Geometry: final body of the model. Coordinates: model frame, mm. A direction names the side the tool comes from. Coordinates: 2 decimals unless noted, no trailing zeros. Order: outer loops, then holes, each group sorted by start corner. A loop starts at its lowest first (then second) coordinate and runs counter-clockwise, first axis right, second up. Notation, with made-up numbers: M -3.75,34.5 L 10.25,34.5 A16 ccw 10.25,62.5 Z; hole C -15,-12 d7. An arc over 180 degrees is marked long. One line per question, with ' | ' between items.
from build123d import *

# Parameters (mm, degrees)
BOSS_EXTRUDE2_DEPTH = 40
SKETCH4_R           = 12
CUT_EXTRUDE4_DEPTH  = 2
SKETCH5_R           = 6
CUT_EXTRUDE5_DEPTH  = 77.576758876
SKETCH6_R           = 3.4
CUT_EXTRUDE6_DEPTH  = 76.498344353
SKETCH7_R           = 3.4
CUT_EXTRUDE7_DEPTH  = 87.394444266


with BuildPart() as part:
    # Sketch1 → Boss-Extrude2 (new body)
    with BuildSketch(Plane(origin=(0, 0, 0), x_dir=(0, 0, -1), z_dir=(1, 0, 0))):
        Polygon((0, 0), (-50, 0), (-50, 18), (0, 18), (0, 58), (14, 58), (14, 0), align=None)
    extrude(amount=BOSS_EXTRUDE2_DEPTH)

    # Sketch4 → Cut-Extrude4 (cut)
    with BuildSketch(Plane(origin=(0, 18, 0), x_dir=(1, 0, 0), z_dir=(0, 1, 0))):
        with Locations(Location((20, -25, 0), (0, 0, 270))):
            Circle(SKETCH4_R)
    extrude(amount=-CUT_EXTRUDE4_DEPTH, mode=Mode.SUBTRACT)

    # Sketch5 → Cut-Extrude5 (cut, through all)
    with BuildSketch(Plane(origin=(0, 16, 0), x_dir=(1, 0, 0), z_dir=(0, 1, 0))):
        with Locations(Location((20, -25, 0), (0, 0, 270))):
            Circle(SKETCH5_R)
    extrude(amount=-CUT_EXTRUDE5_DEPTH, mode=Mode.SUBTRACT)

    # Sketch6 → Cut-Extrude6 (cut, through all)
    with BuildSketch(Plane(origin=(0, 18, 0), x_dir=(1, 0, 0), z_dir=(0, 1, 0))):
        with Locations(Location((20, -9, 0), (0, 0, 270))):
            Circle(SKETCH6_R)
        with Locations(Location((36, -25, 0), (0, 0, 270))):
            Circle(SKETCH6_R)
        with Locations(Location((20, -41, 0), (0, 0, 270))):
            Circle(SKETCH6_R)
        with Locations(Location((4, -25, 0), (0, 0, 270))):
            Circle(SKETCH6_R)
    extrude(amount=-CUT_EXTRUDE6_DEPTH, mode=Mode.SUBTRACT)

    # Sketch7 → Cut-Extrude7 (cut, through all)
    with BuildSketch(Plane.XY):
        with Locations((20, 47)):
            Circle(SKETCH7_R)
        with Locations((32, 35)):
            Circle(SKETCH7_R)
        with Locations((20, 23)):
            Circle(SKETCH7_R)
        with Locations((8, 35)):
            Circle(SKETCH7_R)
    extrude(amount=-CUT_EXTRUDE7_DEPTH, mode=Mode.SUBTRACT)


solid = part.part
1. Pin query (flat end, axial travel): P1, Ø12, axis at x = 20.5, z = 8.5, coming from the +Y side; P2, Ø12, axis at x = 18, y = 35.5, coming from the +Z side; P3, Ø12, axis at x = 24.5, z = 28.5, coming from the +Y side. Return the tip coordinate at first contact, or that it passes through.
Response values:
P1: stops at y = 18 | P2: stops at z = 0 | P3: stops at y = 16
2. Draft query along X for faces 3 (the face through (40, 17, 10)), 4 (the face through (20, 29, -14)), 5 (the face through (18, 16, 19)). Return one class per face: pulls with the +X half, pulls with the -X half, needs draft (parallel to the pull), parting line crosses it, or undercut.
Response values:
face 3: pulls with the +X half | face 4: needs draft | face 5: undercut
3. Section B-B, the plane x = 20. Give the number of separate pieces and of enclosed holes in the cut face, and give its area (3 significant figures).
Response values:
separate pieces: 6 | enclosed holes: 0 | area: 1,040 mm^2
4. Section C-C, the plane z = 41. Output: boundary loops of the cut face in (x, y).
Response values:
outline: M 0,0 L 16.6,0 L 16.6,18 L 0,18 Z; M 23.4,0 L 40,0 L 40,18 L 23.4,18 Z
5. Section A-A, the plane y = 35. Output: boundary loops of the cut face in (x, z), and give its area (3 significant figures).
Response values:
outline: M 0,-14 L 4.6,-14 L 4.6,0 L 0,0 Z; M 11.4,-14 L 28.6,-14 L 28.6,0 L 11.4,0 Z; M 35.4,-14 L 40,-14 L 40,0 L 35.4,0 Z | area: 370 mm^2
6. Access query for faces 1 (the face through (15.3, 18, 36.5)), 2 (the face through (20, 8, 19)). Directions: +Z, -Z, +X, -X, +Y, -Y. A direction counts if a zero-diameter tool reaches every point of the face in a straight line with its end or side. Return the directions, or none.
Response values:
face 1: +Z, +X, -X, +Y | face 2: +Y, -Y
7. Material intervals for line 1 (X direction, y = 16.9, z = 25); line 2 (X direction, y = 5.5, z = 25); line 3 (Y direction, x = 8, z = -9), sorted ascending. Write a range as [from, to].
Response values:
line 1: x = [0, 0.6], [7.4, 8], [32, 32.6], [39.4, 40] | line 2: x = [0, 0.6], [7.4, 14], [26, 32.6], [39.4, 40] | line 3: y = [0, 31.6], [38.4, 58]
8. Section D-D, the plane z = -1. Output: boundary loops of the cut face in (x, y), and give its area (3 significant figures).
Response values:
outline: M 0,0 L 40,0 L 40,58 L 0,58 Z; hole C 8,35 d6.8; hole C 20,23 d6.8; hole C 20,47 d6.8; hole C 32,35 d6.8 | area: 2,170 mm^2
